Geometry check sheet. Reference: drawing and pictorial views, mm from the part's lowest x, y, z. A direction names the side the tool comes from. Coordinates: 2 decimals unless noted, no trailing zeros. Write each loop counter-clockwise with the first axis right and the second up, starting at its lowest first coordinate (ties: lowest second). Pieces come first, ordered by that corner, then holes. Notation, with made-up numbers: (-39, -5.5) -> (18, -5.5) arc R33 ccw to (18, 31.5) -> close; hole circle Ø2 at (-15.5, -5). An arc over 180 degrees is marked (long way). Put each result on its own line as item: value.
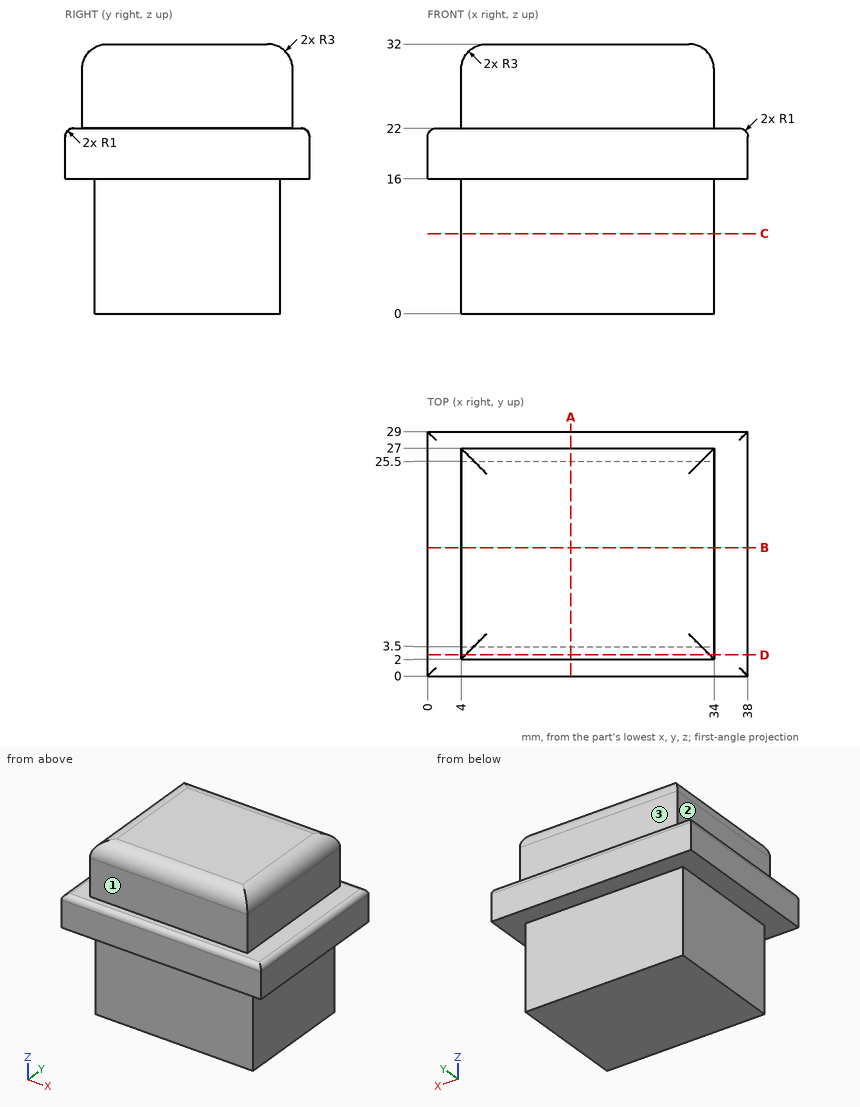
Q1. Cross-section at A-A (x = 17). Record the cut outline in (y, z).
Recorded:
outline: (0, 16) -> (3.5, 16) -> (3.5, 0) -> (25.5, 0) -> (25.5, 16) -> (29, 16) -> (29, 21) arc R1 ccw to (28, 22) -> (27, 22) -> (27, 29) arc R3 ccw to (24, 32) -> (5, 32) arc R3 ccw to (2, 29) -> (2, 22) -> (1, 22) arc R1 ccw to (0, 21) -> close
Q2. Tool access check on the marked faces 1, 2 and 3. Record the directions out of +Z, -Z, +X, -X, +Y, -Y that give a thin tool (end or side, any length) a straight path to the whole face; none if there is none.
Recorded:
face 1: +Z, +X, -X, -Y
face 2: +Z, -X, +Y, -Y
face 3: +Z, +X, -X, +Y
Q3. Material ranges on line 1 along X through (y, z) = (20.25, 24); line 2 along Y through (x, z) = (11, 15); line 3 along Y through (x, z) = (25.5, 28.5), recorded low to high.
Recorded:
line 1: x = 4 to 34
line 2: y = 3.5 to 25.5
line 3: y = 2 to 27
Q4. Depth check by flat-ended pin: P1, Ø5, axis at y = 12.5, z = 9, coming from the -X side; P2, Ø3, axis at x = 16.5, z = 11.5, coming from the +Y side; P3, Ø8, axis at x = 24, z = 7.5, coming from the -Y side. Enter the tip coordinate at first touch or a pass-through.
Recorded:
P1: stops at x = 4
P2: stops at y = 25.5
P3: stops at y = 3.5
Q5. Cross-section at B-B (y = 15.25). Record the cut outline in (x, z).
Recorded:
outline: (0, 16) -> (4, 16) -> (4, 0) -> (34, 0) -> (34, 16) -> (38, 16) -> (38, 21) arc R1 ccw to (37, 22) -> (34, 22) -> (34, 29) arc R3 ccw to (31, 32) -> (7, 32) arc R3 ccw to (4, 29) -> (4, 22) -> (1, 22) arc R1 ccw to (0, 21) -> close
Q6. Cross-section at C-C (z = 9.5). Record the cut outline in (x, y).
Recorded:
outline: (4, 3.5) -> (34, 3.5) -> (34, 25.5) -> (4, 25.5) -> close
Q7. Cross-section at D-D (y = 2.5). Record the cut outline in (x, z), plus the area to 3 significant figures.
Recorded:
outline: (0, 16) -> (38, 16) -> (38, 21) arc R1 ccw to (37, 22) -> (34, 22) -> (34, 29) arc R3 ccw to (33.5, 30.66) -> (4.5, 30.66) arc R3 ccw to (4, 29) -> (4, 22) -> (1, 22) arc R1 ccw to (0, 21) -> close
area: 487 mm2
